The model under review builds one solid part; all positions refer to its coordinate system, in mm. A direction names the side the tool comes from. Round coordinates to 2 decimals unless told otherwise and drop trailing zeros. Loops run counter-clockwise (first coordinate to the right, second up) from the corner with the lowest first, then second, coordinate; pieces in that order, holes last. Notation, with made-up numbers: (34.25, -34) -> (89.25, -34) arc R19 cw to (89.25, -18) -> close; hole circle Ø3 at (-17, -5). An arc over 180 degrees is marked (long way). Use CSV: the item, a comma, the result in double quotes. Start each with the question number.
```python
from build123d import *

# Parameters (mm, degrees)
CROQUIS1_W              = 100
CROQUIS1_H              = 100
SALIENTE_EXTRUIR1_DEPTH = 15
CROQUIS2_R              = 30
CROQUIS2_R_2            = 5
CORTAR_EXTRUIR1_DEPTH   = 15
CROQUIS9_R              = 35
CROQUIS9_R_2            = 30
CROQUIS12_W             = 100
CROQUIS12_H             = 100
SALIENTE_EXTRUIR2_DEPTH = 15
CORTAR_EXTRUIR2_START   = 15
CROQUIS13_R             = 30
CROQUIS13_R_2           = 5
CORTAR_EXTRUIR2_DEPTH   = 15
REDONDEO1_R             = 15


with BuildPart() as part:
    # Croquis1 → Saliente-Extruir1 (new body)
    with BuildSketch(Plane.XY):
        Rectangle(CROQUIS1_W, CROQUIS1_H)
    extrude(amount=SALIENTE_EXTRUIR1_DEPTH)

    # Croquis2 → Cortar-Extruir1 (cut)
    with BuildSketch(Plane.XY):
        Circle(CROQUIS2_R)
        with Locations((-37.5, 37.5)):
            Circle(CROQUIS2_R_2)
        with Locations((37.5, 37.5)):
            Circle(CROQUIS2_R_2)
        with Locations((37.5, -37.5)):
            Circle(CROQUIS2_R_2)
        with Locations((-37.5, -37.5)):
            Circle(CROQUIS2_R_2)
    extrude(amount=CORTAR_EXTRUIR1_DEPTH, mode=Mode.SUBTRACT)

    # Barrer1: sweep along a path in Croquis3
    with BuildLine(Plane(origin=(0, 0, 0), x_dir=(1, 0, 0), z_dir=(0, 1, 0))) as barrer1_path:
        Line((0, 0), (0, 44.08116908))
        ThreePointArc((0, 44.08116908), (10.276263111, 95.743432449), (39.54058454, 139.54058454))
        Line((39.54058454, 139.54058454), (70.710678119, 170.710678119))
    # Croquis9 → Barrer1 (sweep)
    with BuildSketch(Plane.XY):
        Circle(CROQUIS9_R)
        Circle(CROQUIS9_R_2, mode=Mode.SUBTRACT)
    sweep(path=barrer1_path.line)

    # Croquis12 → Saliente-Extruir2 (add)
    with BuildSketch(Plane(origin=(120.710678119, 0, -120.710678119), x_dir=(-0.7071067811865462, 0, -0.7071067811865489), z_dir=(0.7071067811865489, 0, -0.7071067811865462))):
        with Locations((70.710678119, 0)):
            Rectangle(CROQUIS12_W, CROQUIS12_H)
    extrude(amount=SALIENTE_EXTRUIR2_DEPTH)

    # Croquis13 → Cortar-Extruir2 (cut)
    with BuildSketch(Plane(origin=(120.710678119, 0, -120.710678119), x_dir=(-0.7071067811865462, 0, -0.7071067811865489), z_dir=(0.7071067811865489, 0, -0.7071067811865462)).offset(CORTAR_EXTRUIR2_START)):
        with Locations((70.710678119, 0)):
            Circle(CROQUIS13_R)
        with Locations((108.210678119, 37.5)):
            Circle(CROQUIS13_R_2)
        with Locations((108.210678119, -37.5)):
            Circle(CROQUIS13_R_2)
        with Locations((33.210678119, -37.5)):
            Circle(CROQUIS13_R_2)
        with Locations((33.210678119, 37.5)):
            Circle(CROQUIS13_R_2)
    extrude(amount=-CORTAR_EXTRUIR2_DEPTH, mode=Mode.SUBTRACT)

    # Redondeo1
    redondeo1_edges = [part.edges().sort_by_distance(p)[0] for p in [
        (40.658639918, -50, -211.369318037),
        (40.658639918, 50, -211.369318037),
        (111.369318037, 50, -140.658639918),
        (111.369318037, -50, -140.658639918),
        (50, -50, 7.5),
        (-50, -50, 7.5),
        (-50, 50, 7.5),
        (50, 50, 7.5),
    ]]
    fillet(redondeo1_edges, radius=REDONDEO1_R)


solid = part.part
```
1. For faces 1 (the face through (45.49, 45.72, 7.6)), 2 (the face through (45.49, -45.72, 7.6)), 3 (the face through (32.505, -37.28, 7.395)), 4 (the face through (0, -50, 7)), list the 3-axis set-ups (+Z, -Z, +X, -X, +Y, -Y) from which the entire face can be reached by the end or side of a thin tool; tool diameter is ignored.
2. For line 1 along X through (y, z) = (-37, 4); line 2 along Y through (x, z) = (37.5, 9.25), list the stretches that pass through material, from the lowest coordinate up. Write a range as from..to.
3. Clearance check with flat-ended pins moving along their axes: P1, Ø2, axis at x = 21.5, z = -156, coming from the +Y side; P2, Ø12, axis at x = -24.5, y = 7, coming from the -Z side; P3, Ø8, axis at x = -37.5, y = -37.5, coming from the +Z side (3 decimals); P4, Ø2, axis at x = -24.5, z = -78, coming from the -Y side. State where each tip first meets the part, or that it passes through.
4. The part is to be moulded in two halves that separate along X. For faces 5 (the face through (49.979, 34.168, -160.709)), 6 (the face through (-50, 0, 7)), 7 (the face through (-34, 12, 0)), say which applies: pulls with the +X half, pulls with the -X half, needs draft (parallel to the pull), parting line crosses it, or undercut.
5. Take a section at C-C, the plane y = 37.5. Give the boundary of the cut face in (x, z).
6. Take a section at B-B, the plane x = -37.5. Give the boundary of the cut face in (y, z), then the cut area to 3 significant figures.
7. Take a section at D-D, the plane z = -16. Give the boundary of the cut face in (x, y), then the cut area to 3 significant figures.
8. Take a section at A-A, the plane y = -19.5. Give the boundary of the cut face in (x, z).
Results:
1,face 1,"+Z, +X, +Y"
1,face 2,"+Z, +X, -Y"
1,face 3,"+Z"
1,face 4,"+Z, -Z, +X, -X, -Y"
2,line 1,"-49.87..-42.47, -32.53..32.53, 42.47..49.87"
2,line 2,"-49.79..-42.5, -32.5..32.5, 42.5..49.79"
3,P1,"y = 26.03"
3,P2,"z = -115.75"
3,P3,"through"
3,P4,"y = -22.19"
4,face 5,"undercut"
4,face 6,"pulls with the -X half"
4,face 7,"needs draft"
5,outline,"(-49.79, 0) -> (-42.5, 0) -> (-42.5, 15) -> (-49.79, 15) -> close; (-32.5, 0) -> (32.5, 0) -> (32.5, 15) -> (-32.5, 15) -> close; (35.5, -205.92) -> (46.11, -216.52) -> (51.27, -211.37) -> (40.66, -200.76) -> close; (42.5, 0) -> (49.79, 0) -> (49.79, 15) -> (42.5, 15) -> close; (47.73, -193.69) -> (58.34, -204.3) -> (104.3, -158.34) -> (93.69, -147.73) -> close; (100.76, -140.66) -> (111.37, -151.27) -> (116.52, -146.11) -> (105.92, -135.5) -> close"
6,outline,"(-49.79, 0) -> (-42.5, 0) -> (-42.5, 15) -> (-49.79, 15) -> close; (-32.5, 0) -> (32.5, 0) -> (32.5, 15) -> (-32.5, 15) -> close; (42.5, 0) -> (49.79, 0) -> (49.79, 15) -> (42.5, 15) -> close"
6,area,"1,190 mm²"
7,outline,"circle Ø70 at (0, 0); hole circle Ø60 at (0, 0)"
7,area,"1,020 mm²"
8,outline,"(-50, 0) -> (-29.06, 0) -> (-29.06, -44.08) arc R164.06 ccw to (18.99, -160.09) -> (50.16, -191.26) -> (35.36, -206.07) -> (45.96, -216.67) -> (65.2, -197.44) -> (23.42, -155.66) arc R157.8 cw to (-22.8, -44.08) -> (-22.8, 15) -> (-50, 15) -> close; (22.8, -44.08) arc R112.2 ccw to (55.66, -123.42) -> (97.44, -165.2) -> (116.67, -145.96) -> (106.07, -135.36) -> (91.26, -150.16) -> (60.09, -118.99) arc R105.94 cw to (29.06, -44.08) -> (29.06, 0) -> (50, 0) -> (50, 15) -> (22.8, 15) -> close"
